```python
from build123d import *

# Parameters (mm, degrees)
SKETCH1_W           = 7.5
SKETCH1_H           = 5
BOSS_EXTRUDE1_DEPTH = 5


with BuildPart() as part:
    # Sketch1 → Boss-Extrude1 (new body)
    with BuildSketch(Plane.XY):
        Polygon((480, 177.5), (485, 177.5), (485, 187.5), (480, 187.5), (480, 190), (472.5, 190), (472.5, 195), (480, 195), (480, 200), (447.5, 200), (447.5, 195), (377.5, 195), (377.5, 200), (337.5, 200), (337.5, 195), (305, 195), (305, 190), (295, 190), (295, 195), (280, 195), (280, 190), (270, 190), (270, 195), (217.5, 195), (217.5, 200), (177.5, 200), (177.5, 195), (107.5, 195), (107.5, 200), (75, 200), (75, 195), (75, 187.5), (70, 187.5), (70, 177.5), (75, 177.5), (75, 170), (480, 170), align=None)
        with Locations((453.75, 192.5)):
            Rectangle(SKETCH1_W, SKETCH1_H, mode=Mode.SUBTRACT)
    extrude(amount=BOSS_EXTRUDE1_DEPTH)


solid = part.part
```
Work out the finished part from the listing and answer in its coordinate system (mm). Coordinates: 2 decimals unless noted, no trailing zeros. Loops run counter-clockwise (first coordinate to the right, second up) from the corner with the lowest first, then second, coordinate; pieces in that order, holes last. Notation, with made-up numbers: (-1, 13.5) - (3, 13.5) arc R7 cw to (3, 22.5) - close; hole circle Ø2 at (60, 84). An arc over 180 degrees is marked (long way). Use a Markdown table: item, result.
Item 1: Find section A-A, the plane x = 300.5. Determine the outline of the cut face in (y, z), and give its area (3 significant figures).
Evaluation:
| item | result |
|---|---|
| outline | (170, 0) - (190, 0) - (190, 5) - (170, 5) - close |
| area | 100 mm2 |
Item 2: Find section B-B, the plane x = 136. Determine the outline of the cut face in (y, z), and give its area (3 significant figures).
Evaluation:
| item | result |
|---|---|
| outline | (170, 0) - (195, 0) - (195, 5) - (170, 5) - close |
| area | 125 mm2 |
Item 3: Given pin 1 Ø1.5 at (y, z) = (196.5, 2.5) entering from +X; pin 2 Ø2.5 at (x, z) = (482.5, 3.5) entering from +Y; pin 3 Ø1.5 at (x, z) = (301.5, 2) entering from +Y, each flat-ended and moving along its own axis, determine where each tip first touches the part or whether it passes through.
Evaluation:
| item | result |
|---|---|
| pin 1 | stops at x = 480 |
| pin 2 | stops at y = 187.5 |
| pin 3 | stops at y = 190 |
Item 4: Consider probe 1 along X at (y, z) = (196, 1.3); probe 2 along X at (y, z) = (191.75, 2.7); probe 3 along Y at (x, z) = (451.5, 2.95). Determine where each line is inside the solid, lowest interval first. Write a range as from..to.
Evaluation:
| item | result |
|---|---|
| probe 1 | x = 75..107.5, 177.5..217.5, 337.5..377.5, 447.5..480 |
| probe 2 | x = 75..270, 280..295, 305..450, 457.5..472.5 |
| probe 3 | y = 170..190, 195..200 |
